Geometry: see drawing. Coordinates: mm, zero at the bounding-box minimum. A direction names the side the tool comes from. Coordinates: 2 decimals unless noted, no trailing zeros. Loops run counter-clockwise (first coordinate to the right, second up) from the corner with the lowest first, then second, coordinate; pieces in that order, holes last. Notation, with made-up numbers: M 35,42.25 L 92,42.25 A19 cw 92,48.25 Z; hole C 26,3 d5. An arc over 180 degrees is marked long. One line per question, with ' | ' between items. Start each with the question number.
1. Pin query (flat end, axial travel): P1, Ø10, axis at x = 19.5, y = 230.5, coming from the -Z side; P2, Ø6, axis at x = 18.5, y = 285, coming from the +Z side (1 decimal); P3, Ø1.5, axis at y = 199, z = 6, coming from the +X side (1 decimal); P4, Ø4, axis at y = 11.11, z = 14.29, coming from the +X side. Return the tip coordinate at first contact, or that it passes through.
2. Section query B-B, the plane z = 8. Output: boundary loops of the cut face in (x, y) (1 decimal), and give its area (3 significant figures).
3. Section query C-C, the plane x = 19.75. Output: boundary loops of the cut face in (y, z) (1 decimal), and give its area (3 significant figures).
4. Section query A-A, the plane y = 299. Output: boundary loops of the cut face in (x, z) (1 decimal).
5. Access query for the marked faces 1 and 2. Directions: +Z, -Z, +X, -X, +Y, -Y. A direction counts if a zero-diameter tool reaches every point of the face in a straight line with its end or side. Return the directions, or none.
6. Ray query, probe 1 along Z at (x, y) = (20, 242.5) (1 decimal). Return the intervals inside material, ascending.
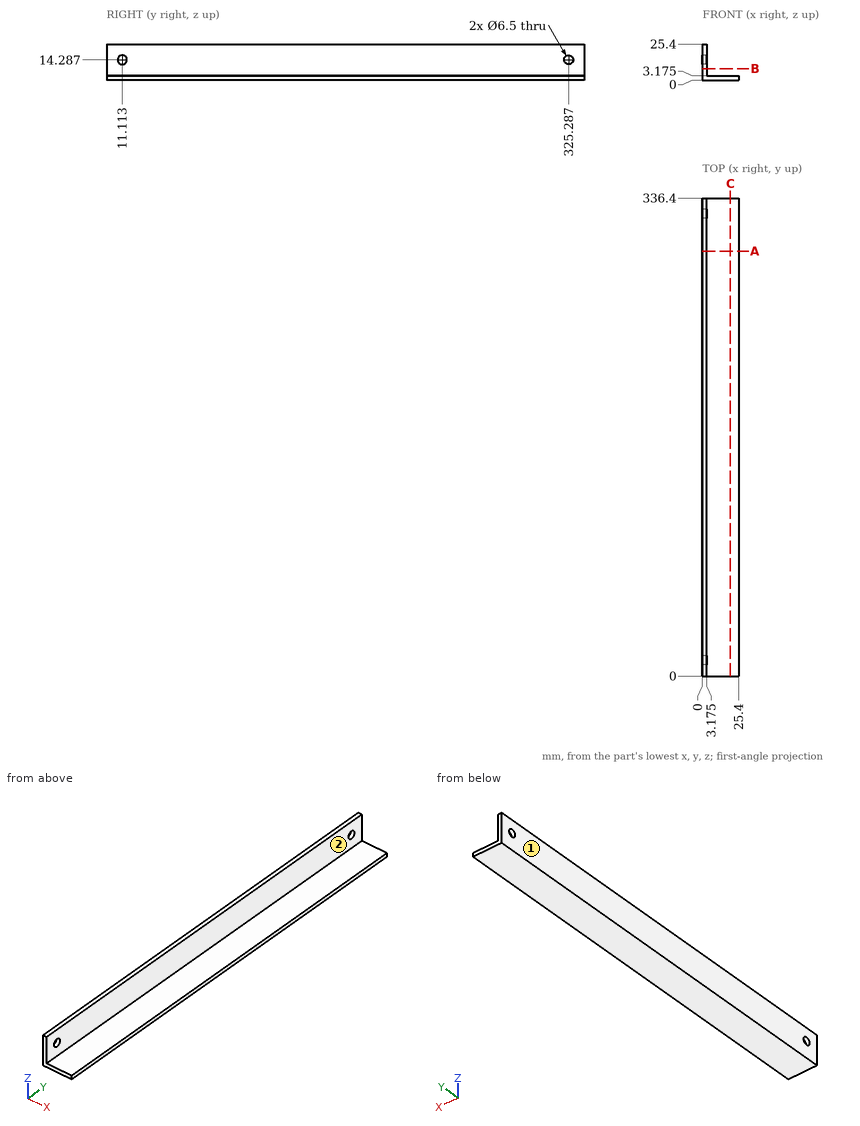
Taken from the geometry:
1) P1: z = 0 | P2: z = 3.2 | P3: x = 3.2 | P4: through
2) outline: M 0,0 L 3.2,0 L 3.2,336.4 L 0,336.4 Z | area: 1,070 mm^2
3) outline: M 0,0 L 336.4,0 L 336.4,3.2 L 0,3.2 Z | area: 1,070 mm^2
4) outline: M 0,0 L 25.4,0 L 25.4,3.2 L 3.2,3.2 L 3.2,25.4 L 0,25.4 Z
5) face 1: +Z, -Z, -X, +Y, -Y | face 2: +Z, +X, +Y, -Y
6) probe 1: 0 to 3.2
